from build123d import *

# Parameters (mm, degrees)
SKETCH1_W                      = 623.5
SKETCH1_H                      = 15
BASE_FLANGE2_DEPTH             = 0.75
EDGE_FLANGE1_STRIP_W           = 13
EDGE_FLANGE1_STRIP_H           = 0.75
EDGE_FLANGE1_STRIP_CUT_DEPTH   = 15
EDGE_FLANGE1_STRIP_2_W         = 13
EDGE_FLANGE1_STRIP_2_H         = 0.75
EDGE_FLANGE1_STRIP_CUT_2_DEPTH = 15
EDGE_FLANGE1_DEPTH             = 15
EDGE_FLANGE1_BEND_DEPTH        = 15
SKETCH17_R                     = 2.5
CUT_EXTRUDE1_DEPTH             = 638.421563802


# Sheet-metal steps are written as plain solids
with BuildPart() as part:
    # Sketch1 → Base-Flange2 (new body)
    with BuildSketch(Plane(origin=(0, 0, 0), x_dir=(1, 0, 0), z_dir=(0, 1, 0))):
        Rectangle(SKETCH1_W, SKETCH1_H)
    extrude(amount=-BASE_FLANGE2_DEPTH)

    # Edge-Flange1 strip (across the edge) → Edge-Flange1 strip cut (cut)
    with BuildSketch(Plane(origin=(311.75, -0.75, -7.5), x_dir=(-1, 0, 0), z_dir=(0, 0, 1))):
        with Locations((-1.5, -0.375)):
            Rectangle(EDGE_FLANGE1_STRIP_W, EDGE_FLANGE1_STRIP_H)
    extrude(amount=EDGE_FLANGE1_STRIP_CUT_DEPTH, mode=Mode.SUBTRACT)

    # Edge-Flange1 strip 2 (across the edge) → Edge-Flange1 strip cut 2 (cut)
    with BuildSketch(Plane(origin=(-311.75, -0.75, 7.5), x_dir=(1, 0, 0), z_dir=(0, 0, -1))):
        with Locations((-1.5, -0.375)):
            Rectangle(EDGE_FLANGE1_STRIP_2_W, EDGE_FLANGE1_STRIP_2_H)
    extrude(amount=EDGE_FLANGE1_STRIP_CUT_2_DEPTH, mode=Mode.SUBTRACT)

    # Edge-Flange1 section (across the edge) → Edge-Flange1 (add)
    with BuildSketch(Plane(origin=(311.75, -0.75, -7.5), x_dir=(-1, 0, 0), z_dir=(0, 0, 1))):
        with BuildLine():
            Line((-0.75, 5), (-0.75, 124.25))
            Line((-0.75, 124.25), (0, 124.25))
            Line((0, 124.25), (0, 5))
            ThreePointArc((0, 5), (1.464466094, 1.464466094), (5, 0))
            Line((5, 0), (5, -0.75))
            ThreePointArc((5, -0.75), (0.934136008, 0.934136008), (-0.75, 5))
        make_face()
    extrude(amount=EDGE_FLANGE1_DEPTH)

    # Edge-Flange1 section 2 (across the edge) → Edge-Flange1 bend (add)
    with BuildSketch(Plane(origin=(-311.75, -0.75, 7.5), x_dir=(1, 0, 0), z_dir=(0, 0, -1))):
        with BuildLine():
            Line((-0.75, 5), (-0.75, 124.25))
            Line((-0.75, 124.25), (0, 124.25))
            Line((0, 124.25), (0, 5))
            ThreePointArc((0, 5), (1.464466094, 1.464466094), (5, 0))
            Line((5, 0), (5, -0.75))
            ThreePointArc((5, -0.75), (0.934136008, 0.934136008), (-0.75, 5))
        make_face()
    extrude(amount=EDGE_FLANGE1_BEND_DEPTH)

    # Sketch17 → Cut-Extrude1 (cut, through all)
    with BuildSketch(Plane(origin=(312.5, 0, 0), x_dir=(0, 0, -1), z_dir=(1, 0, 0))):
        with Locations(Location((0, -120, 0), (0, 0, 90))):
            Circle(SKETCH17_R)
        with BuildLine():
            Line((-5, -111.286267084), (-5, -120))
            ThreePointArc((-5, -120), (0, -125), (5, -120))
            Line((5, -120), (5, -111.286267084))
            Line((5, -111.286267084), (9.961082892, -108.386663731))
            Line((9.961082892, -108.386663731), (9.961082892, -134.171353008))
            Line((9.961082892, -134.171353008), (-9.961082892, -134.171353008))
            Line((-9.961082892, -134.171353008), (-9.961082892, -108.386663731))
            Line((-9.961082892, -108.386663731), (-5, -111.286267084))
        make_face()
    extrude(amount=-CUT_EXTRUDE1_DEPTH, mode=Mode.SUBTRACT)


solid = part.part
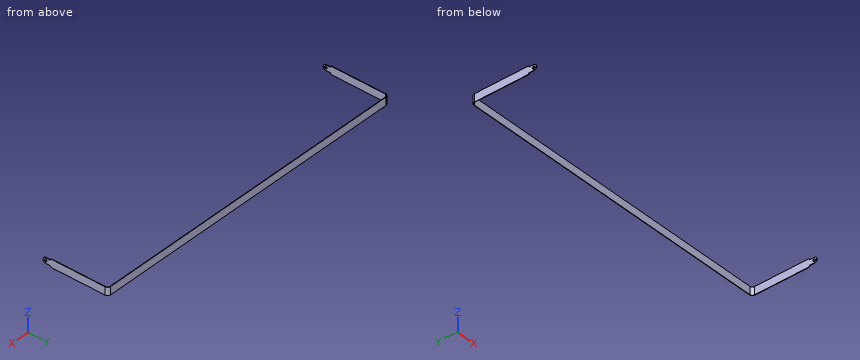
The listing builds one solid part. Answer for the finished solid, in the listing's coordinates (mm). Coordinates: 2 decimals unless noted, no trailing zeros. Loops run counter-clockwise (first coordinate to the right, second up) from the corner with the lowest first, then second, coordinate; pieces in that order, holes last. Notation, with made-up numbers: M 35,61 L 77,61 A22 ccw 77,74 Z; hole C -40,15 d9. An arc over 180 degrees is marked long. Answer in a Markdown table with one row per item.
1) Given pin 1 (8 mm diameter, centred on x = 35, z = 1.5, fed in from +Y); pin 2 (0.8 mm diameter, centred on x = 312, y = -115.5, fed in from +Z); pin 3 (5 mm diameter, centred on x = -110.5, z = 3.5, fed in from -Y); pin 4 (0.6 mm diameter, centred on x = 312, y = -113.5, fed in from -Z), each flat-ended and moving along its own axis, determine where each tip first touches the part or whether it passes through.
Answers below:
| item | result |
|---|---|
| pin 1 | y = 0 |
| pin 2 | z = 5 |
| pin 3 | y = -0.75 |
| pin 4 | z = -5 |
2) Find the intervals of material crossed by probe 1 along X at (y, z) = (-76.5, -3); probe 2 along Z at (x, y) = (-312.15, -120); probe 3 along Y at (x, z) = (174, -1.5), in increasing order.
Answers below:
| item | result |
|---|---|
| probe 1 | -312.5 to -311.75, 311.75 to 312.5 |
| probe 2 | -5 to -2.5, 2.5 to 5 |
| probe 3 | -0.75 to 0 |
3) Find section C-C (x = 3). Determine the outline of the cut face in (y, z).
Answers below:
| item | result |
|---|---|
| outline | M -0.75,-7.5 L 0,-7.5 L 0,7.5 L -0.75,7.5 Z |
4) Find section A-A (y = -75). Determine the outline of the cut face in (x, z).
Answers below:
| item | result |
|---|---|
| outline | M -312.5,-7.5 L -311.75,-7.5 L -311.75,7.5 L -312.5,7.5 Z; M 311.75,-7.5 L 312.5,-7.5 L 312.5,7.5 L 311.75,7.5 Z |
5) Find section B-B (z = 0). Determine the outline of the cut face in (x, y).
Answers below:
| item | result |
|---|---|
| outline | M -312.5,-125 L -311.75,-125 L -311.75,-122.5 L -312.5,-122.5 Z; M -312.5,-117.5 L -311.75,-117.5 L -311.75,-5.75 A5 cw -306.75,-0.75 L 306.75,-0.75 A5 cw 311.75,-5.75 L 311.75,-117.5 L 312.5,-117.5 L 312.5,-5.75 A5.75 ccw 306.75,0 L -306.75,0 A5.75 ccw -312.5,-5.75 Z; M 311.75,-125 L 312.5,-125 L 312.5,-122.5 L 311.75,-122.5 Z |
